Input: part model. Units: mm. Frame: model coordinates. Face numbers are marked on the shaded views. A direction names the side the tool comes from. Give positions to 0.01 mm unless a question says otherwise; leave off trailing zeros. Loops run counter-clockwise (first coordinate to the right, second up) from the corner with the lowest first, then second, coordinate; pieces in that order, holes last.
from build123d import *

# Parameters (mm, degrees)
SKETCH1_R                = 25.4
BOSS_EXTRUDE1_DEPTH      = 88.9
BOSS_EXTRUDE2_DEPTH      = 20.32
BOSS_EXTRUDE2_DEPTH_BACK = 20.32
SKETCH2_W                = 58.42
SKETCH2_H                = 25.4
FILLET1_R                = 12.7
SKETCH3_R                = 12.7
CUT_EXTRUDE3_DEPTH       = 155.272331933


with BuildPart() as part:
    # Sketch1 → Boss-Extrude1 (new body)
    with BuildSketch(Plane.XY):
        Circle(SKETCH1_R)
    extrude(amount=-BOSS_EXTRUDE1_DEPTH)

    # Sketch2 → Boss-Extrude2 (add, two sides: drawn at the far end of the back side and taken through both)
    with BuildSketch(Plane(origin=(0, 0, 0), x_dir=(0, 0, -1), z_dir=(1, 0, 0)).offset(-BOSS_EXTRUDE2_DEPTH_BACK)):
        with Locations((118.11, 0)):
            Rectangle(SKETCH2_W, SKETCH2_H)
    extrude(amount=BOSS_EXTRUDE2_DEPTH + BOSS_EXTRUDE2_DEPTH_BACK)

    # Fillet1
    fillet1_edges = [part.edges().sort_by_distance(p)[0] for p in [
        (-20.32, 0, -147.32),
        (20.32, 0, -147.32),
    ]]
    fillet(fillet1_edges, radius=FILLET1_R)

    # Sketch3 → Cut-Extrude3 (cut, through all)
    with BuildSketch(Plane(origin=(0, 12.7, 0), x_dir=(1, 0, 0), z_dir=(0, 1, 0))):
        with Locations(Location((0, 127, 0), (0, 0, 270))):
            Circle(SKETCH3_R)
    extrude(amount=-CUT_EXTRUDE3_DEPTH, mode=Mode.SUBTRACT)


solid = part.part
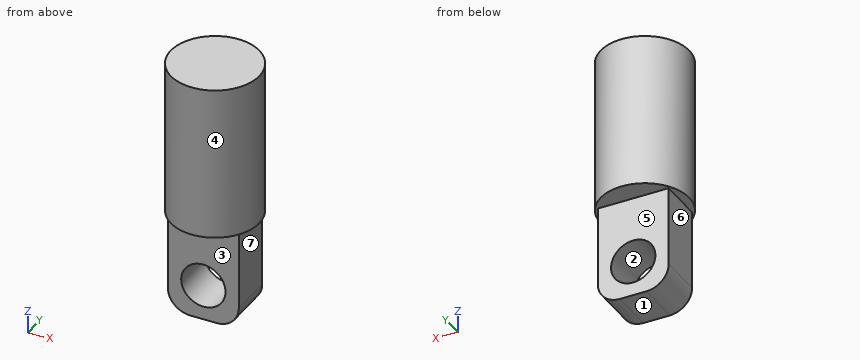
(1) Cut plane A-A (y = 0). Return the cut outline in (x, z).
Values follow:
outline: (-25.4, -88.9) - (-20.32, -88.9) - (-20.32, -134.62) arc R12.7 ccw to (-7.62, -147.32) - (7.62, -147.32) arc R12.7 ccw to (20.32, -134.62) - (20.32, -88.9) - (25.4, -88.9) - (25.4, 0) - (-25.4, 0) - close; hole circle Ø25.4 at (0, -127)
(2) Cut plane B-B (x = 0). Return the cut outline in (y, z).
Values follow:
outline: (-25.4, -88.9) - (-12.7, -88.9) - (-12.7, -114.3) - (12.7, -114.3) - (12.7, -88.9) - (25.4, -88.9) - (25.4, 0) - (-25.4, 0) - close; (-12.7, -147.32) - (12.7, -147.32) - (12.7, -139.7) - (-12.7, -139.7) - close
(3) Reachability of the marked faces 4, 5, 6 and 7 from +Z, -Z, +X, -X, +Y, -Y: full face, straight path, thin tool, end or side. Return the list, or none.
Values follow:
face 4: +Z, -Z
face 5: -Z, +X, -X, +Y
face 6: -Z, -X, +Y, -Y
face 7: -Z, +X, +Y, -Y
(4) Pin query (flat end, axial travel): pin 1 Ø1 at (x, y) = (-11, 19.5) entering from -Z; pin 2 Ø5 at (x, z) = (-13.5, -38.5) entering from -Y; pin 3 Ø20.5 at (y, z) = (-5.5, -108) entering from +X; pin 4 Ø20.5 at (x, z) = (0, -127) entering from +Y (3 decimals). Return the tip coordinate at first contact, or that it passes through.
Values follow:
pin 1: stops at z = -88.9
pin 2: stops at y = -22.89
pin 3: stops at x = 20.32
pin 4: passes through
(5) Cut plane D-D (z = -79). Return the cut outline in (x, y).
Values follow:
outline: circle Ø50.8 at (0, 0)
(6) Cut plane C-C (z = -127). Return the cut outline in (x, y), and give its area (3 significant figures).
Values follow:
outline: (-20.32, -12.7) - (-12.7, -12.7) - (-12.7, 12.7) - (-20.32, 12.7) - close; (12.7, -12.7) - (20.32, -12.7) - (20.32, 12.7) - (12.7, 12.7) - close
area: 387 mm2
(7) Mould query, pull axis Z, two halves, no side actions, for the marked faces 1, 2 and 3. Classes: +Z half, -Z half, draft (parallel to the pull), parting line (faces both ways), or undercut.
Values follow:
face 1: -Z half
face 2: undercut
face 3: draft
(8) Ray query, probe 1 along X at (y, z) = (-3.25, -127); probe 2 along Z at (x, y) = (8.5, -15); probe 3 along Y at (x, z) = (-18, -112.5). Return the intervals inside material, ascending.
Values follow:
probe 1: x = -20.32 to -12.7, 12.7 to 20.32
probe 2: z = -88.9 to 0
probe 3: y = -12.7 to 12.7
